Autodesk Inventor part; units mm, degrees
ref_plane "YZ Plane" through (0, 0, 0) normal (1, 0, 0) x (0, 1, 0)
ref_plane "XZ Plane" through (0, 0, 0) normal (0, 1, 0) x (-1, 0, 0)
ref_plane "XY Plane" through (0, 0, 0) normal (0, 0, 1) x (1, 0, 0)
sketch "Sketch1" plane through (0, 0, 0) normal (0, 1, 0) x (-1, 0, 0)
  circle A0 centre (0, 0) radius 6.35
  circle A1 centre (0, -101.6) radius 6.35
  line L0 (0, 0) -> (0, -109.4726) construction
  line L1 (6.35, -101.6) -> (6.35, 0)
  line L2 (-6.35, -101.6) -> (-6.35, 0)
  dimension "d0" = 101.6
  dimension "d1" = 12.7
  dimension "d2" = 12.7
extrude "Extrusion1" add sketch "Sketch1" along normal blind 6.35
hole "Hole1" at (0, 0, 0) at (0, 0, -101.6) direction (0, 1, 0) diameter 5.1054 depth 13.6144
chamfer "Chamfer1" [suppressed]
properties part number "Main Linkage"
Check sheet for the modelled part. Datum: model origin and axes. Units: mm. Round coordinates to 2 decimals unless told otherwise and drop trailing zeros. Loops run counter-clockwise (first coordinate to the right, second up) from the corner with the lowest first, then second, coordinate; pieces in that order, holes last. Notation, with made-up numbers: (-11.75, -0.75) - (10.25, -0.75) arc R22 ccw to (10.25, 34.25) - close; hole circle Ø10 at (-5.5, 33.25). An arc over 180 degrees is marked (long way). Answer as CSV lines item,"result". Start each with the question number.
Item 1: Section check B-B (y = 4.75). Record the boundary of the cut face in (x, z), and give its area (3 significant figures).
Item 2: Release check for a two-part mould opening along X. For faces 1 (the flat face through (0, 0, -50)), 2 (the cylindrical face through (0.14, 3.13, 6.35)), 3 (the cylindrical face through (-0.767, 3.219, -104.035)) record: +X half, -X half, draft (parallel to the pull), parting line (faces both ways), or undercut.
Item 3: Section check A-A (x = 0). Record the boundary of the cut face in (y, z), and give its area (3 significant figures).
Item 4: Depth check by flat-ended pin: P1, Ø6.5, axis at x = 0, z = -101.6, coming from the +Y side; P2, Ø1.5, axis at x = 5, y = 2.5, coming from the +Z side; P3, Ø2, axis at x = -1.5, y = 3, coming from the +Z side; P4, Ø4.5, axis at x = 0, z = 0, coming from the -Y side. Enter the tip coordinate at first touch or a pass-through.
Item 5: Scan lines: line 1 (Z direction, x = 0, y = 2.75); line 2 (X direction, y = 4, z = -101.6). Record each from-to range of solid material in increasing order. Write a range as [from, to].
Item 6: Section check D-D (x = -5). Record the boundary of the cut face in (y, z), and give its area (3 significant figures).
Item 7: Section check C-C (x = 4.75). Record the boundary of the cut face in (y, z), and give its area (3 significant figures).
Report:
1,outline,"(-6.35, -101.6) arc R6.35 ccw to (6.35, -101.6) - (6.35, 0) arc R6.35 ccw to (-6.35, 0) - close; hole circle Ø5.11 at (0, -101.6); hole circle Ø5.11 at (0, 0)"
1,area,"1,380 mm2"
2,face 1,"draft"
2,face 2,"parting line"
2,face 3,"undercut"
3,outline,"(0, -107.95) - (6.35, -107.95) - (6.35, -104.15) - (0, -104.15) - close; (0, -99.05) - (6.35, -99.05) - (6.35, -2.55) - (0, -2.55) - close; (0, 2.55) - (6.35, 2.55) - (6.35, 6.35) - (0, 6.35) - close"
3,area,"661 mm2"
4,P1,"stops at y = 6.35"
4,P2,"stops at z = 4.72"
4,P3,"stops at z = 6.33"
4,P4,"passes through"
5,line 1,"z = [-107.95, -104.15], [-99.05, -2.55], [2.55, 6.35]"
5,line 2,"x = [-6.35, -2.55], [2.55, 6.35]"
6,outline,"(0, -105.51) - (6.35, -105.51) - (6.35, 3.91) - (0, 3.91) - close"
6,area,"695 mm2"
7,outline,"(0, -105.81) - (6.35, -105.81) - (6.35, 4.21) - (0, 4.21) - close"
7,area,"699 mm2"
